Design review of the part built by this model. Coordinates are the model's own, in mm. Face numbers are marked on the shaded views. A direction names the side the tool comes from. Round coordinates to 2 decimals unless told otherwise and drop trailing zeros. Order: outer loops, then holes, each group sorted by start corner. A loop starts at its lowest first (then second) coordinate and runs counter-clockwise, first axis right, second up. Notation, with made-up numbers: M -26.75,68.5 L -11.75,68.5 A17 cw -11.75,92.5 Z; hole C 7,72 d5. An arc over 180 degrees is marked long. Use a Markdown table: item, result. Add a question column.
(1) To check wall thickness, follow probe 1 along X at (y, z) = (35, 18); probe 2 along X at (y, z) = (42, 13.5); probe 3 along Z at (x, y) = (-37, 38). State the ranges of each line that lie inside material, in increasing order. Write a range as from..to.
(2) The part is to be moulded in two halves that separate along X. For the marked faces 1, 2, 3 and 4, say which applies: released by +X, released by -X, zero draft, split by the parting line, or undercut.
(3) Take a section at D-D (y = 63). Write out the cut boundary in (x, z).
(4) Take a section at A-A (y = 53.5). Write out the cut boundary in (x, z).
(5) Machinability: for the marked faces 5, 6 and 7, which of the approach directions +Z, -Z, +X, -X, +Y, -Y give a long, thin tool a straight path to every point of the face, cutting with its end or side? Answer none if there is none.
(6) Take a section at C-C (x = -16.5). Write out the cut boundary in (y, z).
(7) Take a section at B-B (z = 56). Write out the cut boundary in (x, y).
(8) For pin 1 (6 mm diameter, centred on x = -53.5, y = 48, fed in from +Z); pin 2 (10 mm diameter, centred on x = -98, y = 56, fed in from +Z); pin 3 (1 mm diameter, centred on x = -34, y = 18.5, fed in from +Z), all flat-tipped, find the tip position at first contact; note any pin that passes through.
```python
from build123d import *

# Parameters (mm, degrees)
BOSS_EXTRUDE1_DEPTH = 74
CUT_EXTRUDE1_DEPTH  = 126
SKETCH3_W           = 30
SKETCH3_H           = 24
CUT_EXTRUDE2_DEPTH  = 48


with BuildPart() as part:
    # Sketch1 → Boss-Extrude1 (new body)
    with BuildSketch(Plane.XY):
        with BuildLine():
            Line((0, 0), (-53.1821954, 0))
            ThreePointArc((-53.1821954, 0), (-80.068712849, 36.611962713), (-125, 29.941125497))
            Line((-125, 29.941125497), (-125, 65.119334087))
            Line((-125, 65.119334087), (-78, 49.848108364))
            Line((-78, 49.848108364), (-26, 73))
            Line((-26, 73), (0, 73))
            Line((0, 73), (0, 0))
        make_face()
    extrude(amount=BOSS_EXTRUDE1_DEPTH)

    # Sketch2 → Cut-Extrude1 (cut, through all)
    with BuildSketch(Plane(origin=(0, 0, 0), x_dir=(0, 0, -1), z_dir=(1, 0, 0))):
        Polygon((-74, 0), (-39.959540955, 73), (-74, 73), align=None)
    extrude(amount=-CUT_EXTRUDE1_DEPTH, mode=Mode.SUBTRACT)

    # Sketch3 → Cut-Extrude2 (cut)
    with BuildSketch(Plane(origin=(-31.426088247, 70.584149863, 0), x_dir=(0.913545458, 0.406736643, 0), z_dir=(-0.406736643, 0.913545458, 0))):
        with Locations((-16.060406954, -23)):
            Rectangle(SKETCH3_W, SKETCH3_H)
    extrude(amount=-CUT_EXTRUDE2_DEPTH, mode=Mode.SUBTRACT)


solid = part.part
```
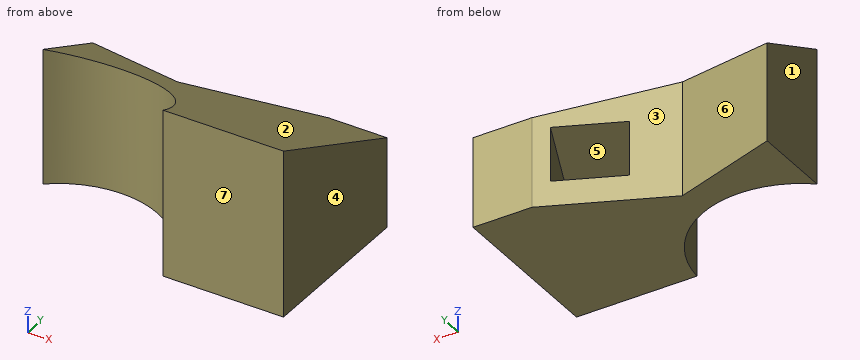
Verdict:
| question | item | result |
|---|---|---|
| 1 | probe 1 | x = -125..-117.37, -76.63..-49.58, -16.74..0 |
| 1 | probe 2 | x = -125..-52.7, -19.86..0 |
| 1 | probe 3 | z = 0..11, 35..56.28 |
| 2 | face 1 | released by -X |
| 2 | face 2 | zero draft |
| 2 | face 3 | undercut |
| 2 | face 4 | released by +X |
| 3 | outline | M -125,0 L -118.48,0 L -118.48,44.62 L -125,44.62 Z; M -48.46,0 L 0,0 L 0,44.62 L -48.46,44.62 L -48.46,35 L -29.21,35 L -29.21,11 L -48.46,11 Z |
| 4 | outline | M -125,0 L -89.24,0 L -89.24,49.05 L -125,49.05 Z; M -69.8,0 L 0,0 L 0,49.05 L -69.8,49.05 Z; hole M -57.82,11 L -24.98,11 L -24.98,35 L -57.82,35 Z |
| 5 | face 5 | none |
| 5 | face 6 | +Z, -Z, +Y |
| 5 | face 7 | +Z, -Z, +X, -X, -Y |
| 6 | outline | M 0,0 L 73,0 L 73,39.96 L 0,74 Z; hole M 24.69,11 L 34.45,11 L 34.45,35 L 24.69,35 Z |
| 7 | outline | M -125,29.94 A44 cw -108.01,38.6 L -125,38.6 Z; M -85.99,38.6 A44 cw -53.18,0 L 0,0 L 0,38.6 Z |
| 8 | pin 1 | stops at z = 53.02 |
| 8 | pin 2 | stops at z = 50.22 |
| 8 | pin 3 | stops at z = 65.61 |
